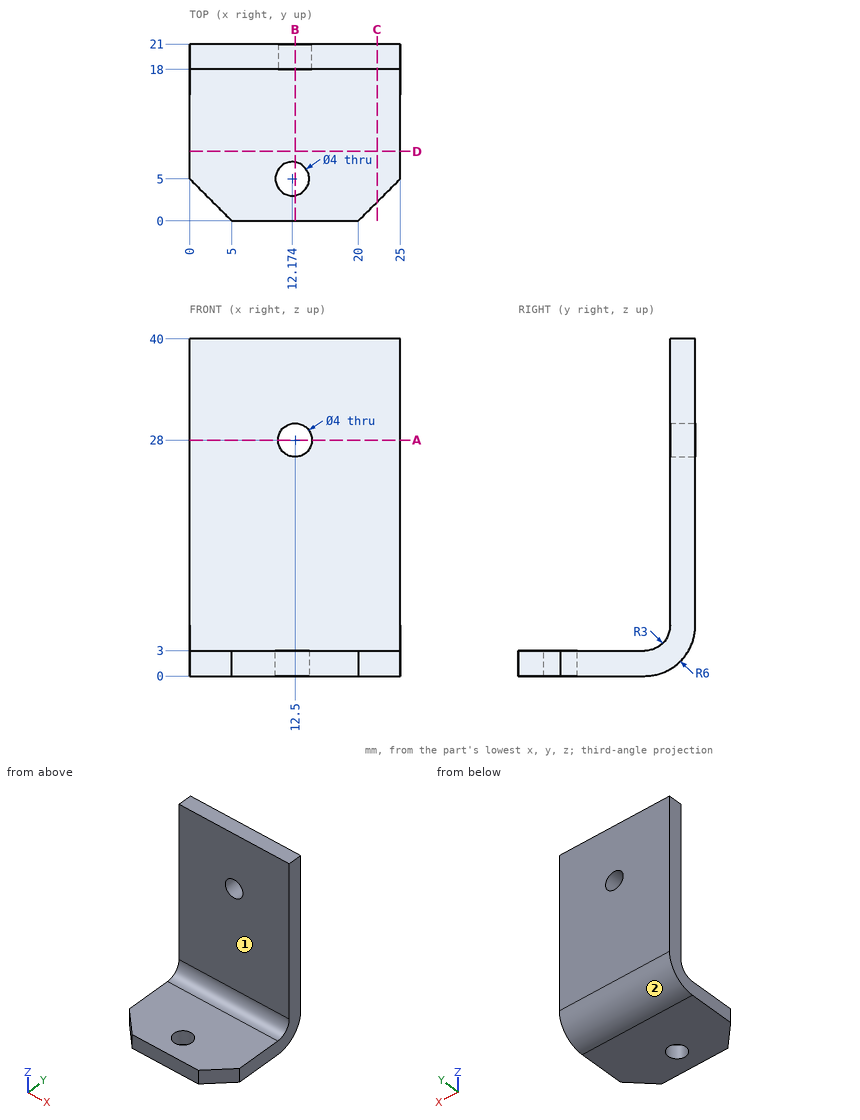
Input: dimensioned drawing with shaded views. Units: mm. Origin: part minimum x, y, z. A direction names the side the tool comes from. Coordinates: 2 decimals unless noted, no trailing zeros. Loops run counter-clockwise (first coordinate to the right, second up) from the corner with the lowest first, then second, coordinate; pieces in that order, holes last. Notation, with made-up numbers: M 2,-3.75 L 45,-3.75 A12 cw 45,18.25 Z; hole C -25,53.5 d9. An arc over 180 degrees is marked long. One line per item, written item: value. Start each with the question number.
1) Cut plane D-D (y = 8.25). Return loops of the section in (x, z), then the cut area to 3 significant figures.
2) Cut plane A-A (z = 28). Return loops of the section in (x, y), then the cut area to 3 significant figures.
3) Cut plane C-C (x = 22.25). Return loops of the section in (y, z).
4) Reachability of the marked faces 1 and 2 from +Z, -Z, +X, -X, +Y, -Y: full face, straight path, thin tool, end or side. Return the list, or none.
5) Cut plane B-B (x = 12.5). Return loops of the section in (y, z).
6) Pin query (flat end, axial travel): P1, Ø12.5, axis at x = 14.5, z = 19, coming from the -Y side; P2, Ø2.5, axis at x = 12.5, z = 28, coming from the -Y side; P3, Ø12, axis at x = 9, y = 8.5, coming from the +Z side. Return the tip coordinate at first contact, or that it passes through.
7) Material intervals for L1, parallel to Z at x = 11.5, y = 13; L2, parallel to Y at x = 12.5, z = 30.5; L3, parallel to Z at x = 11.5, y = 20.25 (1 decimal), sorted ascending. Write a range as from..to.
Evaluation:
1. outline: M 0,0 L 25,0 L 25,3 L 0,3 Z
1. area: 75.0 mm^2
2. outline: M 0,18 L 10.5,18 L 10.5,21 L 0,21 Z; M 14.5,18 L 25,18 L 25,21 L 14.5,21 Z
2. area: 63.0 mm^2
3. outline: M 2.25,0 L 15,0 A6 ccw 21,6 L 21,40 L 18,40 L 18,6 A3 cw 15,3 L 2.25,3 Z
4. face 1: +Z, +X, -X, -Y
4. face 2: -Z, +X, -X, +Y
5. outline: M 0,0 L 3.03,0 L 3.03,3 L 0,3 Z; M 6.97,0 L 15,0 A6 ccw 21,6 L 21,26 L 18,26 L 18,6 A3 cw 15,3 L 6.97,3 Z; M 18,30 L 21,30 L 21,40 L 18,40 Z
6. P1: y = 18
6. P2: through
6. P3: z = 3
7. L1: 0..3
7. L2: 18..21
7. L3: 3.1..26.3, 29.7..40
